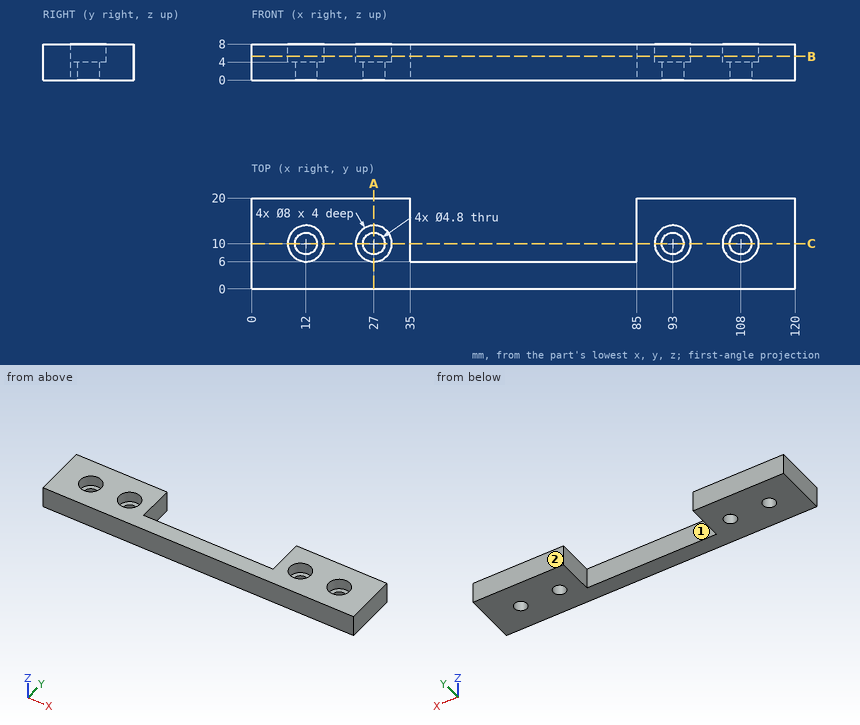
Study the drawing (mm; zero at the part's minimum x, y, z) and answer. Round coordinates to 2 decimals unless told otherwise and drop trailing zeros. Write each loop counter-clockwise with the first axis right and the second up, starting at its lowest first coordinate (ties: lowest second). Pieces come first, ordered by that corner, then holes. Notation, with made-up numbers: (49, 33.5) - (103, 33.5) arc R21 cw to (103, 62.5) - close; hole circle Ø2 at (-0.75, 88). An arc over 180 degrees is marked (long way). Return JSON: item names as keys, results as strings. Group by question number.
Q1. The part is cut by section C-C on y = 10. Count the separate pieces of the cut face and the enclosed holes in it, then the cut area to 3 significant figures.
Q2. The part is cut by section A-A on x = 27. Write down the section's boundary in (y, z), then the cut area to 3 significant figures.
Q3. The part is cut by section B-B on z = 5.25. Write down the section's boundary in (x, y), then the cut area to 3 significant figures.
Q4. The mould has two halves that part along X. Classify the marked faces 1 and 2: released by +X, released by -X, zero draft, split by the parting line, or undercut.
Q5. Each of these flat-tipped pins is pushed along its axis until it touches: pin 1 Ø5 at (x, y) = (12, 10) entering from -Z; pin 2 Ø4 at (x, y) = (93, 11.5) entering from +Z; pin 3 Ø4 at (x, y) = (12, 10) entering from +Z. Where does it stop, or does it pass through?
Q6. Find the intervals of material crossed by L1, parallel to Y at x = 12, z = 6.8; L2, parallel to Y at x = 108, z = 0.8; L3, parallel to X at y = 8.5, z = 4.5, in increasing order.
Solved:
{
 "1": {"separate pieces": "6", "enclosed holes": "0", "area": "355 mm²"},
 "2": {"outline": "(0, 0) - (7.6, 0) - (7.6, 4) - (6, 4) - (6, 8) - (0, 8) - close; (12.4, 0) - (20, 0) - (20, 8) - (14, 8) - (14, 4) - (12.4, 4) - close", "area": "109 mm²"},
 "3": {"outline": "(0, 0) - (120, 0) - (120, 20) - (85, 20) - (85, 6) - (35, 6) - (35, 20) - (0, 20) - close; hole circle Ø8 at (12, 10); hole circle Ø8 at (27, 10); hole circle Ø8 at (93, 10); hole circle Ø8 at (108, 10)", "area": "1,500 mm²"},
 "4": {"face 1": "undercut", "face 2": "zero draft"},
 "5": {"pin 1": "z = 0", "pin 2": "z = 4", "pin 3": "through"},
 "6": {"L1": "0 to 6, 14 to 20", "L2": "0 to 7.6, 12.4 to 20", "L3": "0 to 8.29, 15.71 to 23.29, 30.71 to 35, 85 to 89.29, 96.71 to 104.29, 111.71 to 120"}
}
